Autodesk Inventor part; units mm, degrees
ref_plane "YZ Plane" through (0, 0, 0) normal (1, 0, 0) x (0, 1, 0)
ref_plane "XZ Plane" through (0, 0, 0) normal (0, 1, 0) x (-1, 0, 0)
ref_plane "XY Plane" through (0, 0, 0) normal (0, 0, 1) x (1, 0, 0)
sketch "スケッチ1" plane through (0, 0, 0) normal (1, 0, 0) x (0, 1, 0)
  line L0 (6.25, 11.325) -> (-6.25, 11.325)
  line L1 (-6.25, 11.325) -> (-6.25, -11.325)
  line L2 (-6.25, -11.325) -> (6.25, -11.325)
  line L3 (6.25, -11.325) -> (6.25, 11.325)
  point P0 (0, 0)
  dimension "d0" = 22.65
  dimension "d1" = 12.5
  dimension "d4" = 6.25
  dimension "d5" = 6.25
  dimension "d6" = 11.325
  dimension "d7" = 11.325
extrude "押し出し1" add sketch "スケッチ1" along normal blind 16
sketch "スケッチ2" plane through (16, 0, 0) normal (1, 0, 0) x (0, 0, -1)
  line L0 (-11.325, 6.25) -> (-11.325, -6.25)
  line L1 (-11.325, 6.25) -> (-16.325, 6.25)
  line L2 (-16.325, 6.25) -> (-16.325, -6.25)
  line L3 (-16.325, -6.25) -> (-11.325, -6.25)
  line L4 (-11.325, -6.25) -> (-11.325, 6.25)
  line L5 (11.325, -6.25) -> (11.325, 6.25)
  line L6 (11.325, 6.25) -> (16.325, 6.25)
  line L7 (16.325, 6.25) -> (16.325, -6.25)
  line L8 (16.325, -6.25) -> (11.325, -6.25)
  line L9 (11.325, -6.25) -> (11.325, 6.25)
  circle A0 centre (-13.825, 0) radius 1
  circle A1 centre (13.825, 0) radius 1
  line L10 (-11.325, -6.25) -> (11.325, -6.25)
  line L11 (-11.325, 6.25) -> (11.325, 6.25)
  line L12 (11.325, 6.25) -> (11.325, -6.25)
  line L13 (11.325, -6.25) -> (-11.325, -6.25)
  line L14 (-11.325, -6.25) -> (-11.325, 6.25)
  point P0 (0, 0)
  dimension "d8" = 5
  dimension "d9" = 5
  dimension "d10" = 1.5
  dimension "d11" = 1.5
  dimension "d12" = 2
  dimension "d13" = 2
extrude "押し出し2" add sketch "スケッチ2" along normal blind 2.4
sketch "スケッチ3" plane through (18.4, 0, 0) normal (1, 0, 0) x (0, 0, -1)
  line L0 (-11.325, 6.25) -> (-11.325, -6.25)
  line L1 (11.325, -6.25) -> (16.325, -6.25)
  line L2 (-11.325, 6.25) -> (11.325, 6.25)
  line L3 (11.325, 6.25) -> (11.325, -6.25)
  line L4 (11.325, -6.25) -> (-11.325, -6.25)
  line L5 (-11.325, -6.25) -> (-11.325, 6.25)
  point P0 (0, 0)
extrude "押し出し3" add sketch "スケッチ3" along normal blind 4
sketch "スケッチ4" plane through (22.4, 0, 0) normal (1, 0, 0) x (0, 0, -1)
  circle A0 centre (-5.0802, 0) radius 6.2448
  line L0 (-11.325, 6.25) -> (-11.325, -6.25)
  circle A1 centre (1.0094, 0) radius 1.9656
  circle A2 centre (-5.0802, 0) radius 2.4
  point P0 (0, 0)
  dimension "d18" = 0
  dimension "d19" = 12.4895
  dimension "d20" = 3.9311
  dimension "d21" = 14.3
  dimension "d22" = 4.8
extrude "押し出し4" add sketch "スケッチ4" along normal blind 4.3
sketch "スケッチ5" plane through (22.4, 0, 5.0802) normal (1, 0, 0) x (0, 0, -1)
  circle A0 centre (0, 0) radius 2.4
  point P0 (5.0802, 0)
extrude "押し出し5" add sketch "スケッチ5" along normal blind 7.3
properties part number "microservo"
The listing builds one solid part. Answer for the finished solid, in the listing's coordinates (mm). A direction names the side the tool comes from. Round coordinates to 2 decimals unless told otherwise and drop trailing zeros. Loops run counter-clockwise (first coordinate to the right, second up) from the corner with the lowest first, then second, coordinate; pieces in that order, holes last. Notation, with made-up numbers: (39, -7.75) - (80, -7.75) arc R32 ccw to (80, 31.25) - close; hole circle Ø2 at (0, 28). An arc over 180 degrees is marked (long way). Use one line per item in the form item = value. Start each with the question number.
1. The part is cut by section D-D on z = -6. Determine the outline of the cut face in (x, y), then the cut area to 3 significant figures.
2. The part is cut by section A-A on z = 4. Determine the outline of the cut face in (x, y).
3. Given pin 1 Ø1.5 at (x, z) = (25.5, 5) entering from +Y; pin 2 Ø3 at (y, z) = (0, 13.825) entering from -X; pin 3 Ø4 at (y, z) = (-3, -12.5) entering from +X, each flat-ended and moving along its own axis, determine where each tip first touches the part or whether it passes through.
4. The part is cut by section C-C on x = 20.5. Determine the outline of the cut face in (y, z) (3 decimals).
5. A tool of negligible diameter and unlimited length cuts with its end or side. For faces 1 (the face through (16, 0, -15)), 2 (the face through (18.4, 0, -15)), 3 (the face through (16, 0, 15)), 4 (the face through (24.52, -0.25, 11.32)), 5 (the face through (20, 0, 11.325)), from which of +Z, -Z, +X, -X, +Y, -Y can it reach the whole face along a straight path? Write none if from no direction.
6. The part is cut by section B-B on y = 4.5. Determine the outline of the cut face in (x, z) (3 decimals).
7. Consider line 1 (X direction, y = 1.75, z = 7); line 2 (X direction, y = 3, z = 13); line 3 (Z direction, x = 5.25, y = 5.25) (3 decimals). Determine where each line is inside the solid, lowest interval first. Write a range as [from, to].
8. For a pull along Z with two mould halves and no side action, classify faces 6 (the face through (8, 0, 11.325)), 7 (the face through (17.18, -0.3, 12.87)), 8 (the face through (20, 0, -11.325)) as pulls with the +Z half, pulls with the -Z half, needs draft (parallel to the pull), parting line crosses it, or undercut.
Geometry check:
q1.outline = (0, -6.25) - (22.4, -6.25) - (22.4, 6.25) - (0, 6.25) - close
q1.area = 280 mm^2
q2.outline = (0, -6.25) - (22.4, -6.25) - (22.4, -6.15) - (26.7, -6.15) - (26.7, -2.14) - (29.7, -2.14) - (29.7, 2.14) - (26.7, 2.14) - (26.7, 6.15) - (22.4, 6.15) - (22.4, 6.25) - (0, 6.25) - close
q3.pin_1 = 6.24
q3.pin_2 = 16
q3.pin_3 = 22.4
q4.outline = (-6.25, -11.325) - (6.25, -11.325) - (6.25, 11.325) - (-6.25, 11.325) - close
q5.face_1 = -Z, -X, +Y, -Y
q5.face_2 = -Z, +X, +Y, -Y
q5.face_3 = +Z, -X, +Y, -Y
q5.face_4 = +X
q5.face_5 = +Z, +X, +Y, -Y
q6.outline = (0, -11.325) - (16, -11.325) - (16, -16.325) - (18.4, -16.325) - (18.4, -11.325) - (22.4, -11.325) - (22.4, 0.75) - (26.7, 0.75) - (26.7, 9.41) - (22.4, 9.41) - (22.4, 11.325) - (18.4, 11.325) - (18.4, 16.325) - (16, 16.325) - (16, 11.325) - (0, 11.325) - close
q7.line_1 = [0, 26.7]
q7.line_2 = [16, 18.4]
q7.line_3 = [-11.325, 11.325]
q8.face_6 = pulls with the +Z half
q8.face_7 = undercut
q8.face_8 = pulls with the -Z half
